```python
from build123d import *

# Parameters (mm, degrees)
SKETCH1_R           = 68.2625
SKETCH1_R_2         = 26.9875
BOSS_EXTRUDE1_DEPTH = 3.175


with BuildPart() as part:
    # Sketch1 → Boss-Extrude1 (new body)
    with BuildSketch(Plane.XY):
        Circle(SKETCH1_R)
        Circle(SKETCH1_R_2, mode=Mode.SUBTRACT)
        with BuildLine():
            ThreePointArc((-13.407442068, 58.659886532), (-30.0863, 52.111000212), (-44.097230886, 40.941128696))
            ThreePointArc((-44.097230886, 40.941128696), (-43.930699534, 36.454089884), (-39.443660721, 36.620621236))
            ThreePointArc((-39.443660721, 36.620621236), (-26.9113, 46.611738898), (-11.992557932, 52.46952282))
            ThreePointArc((-11.992557932, 52.46952282), (-9.604818144, 56.272146744), (-13.407442068, 58.659886532))
        make_face(mode=Mode.SUBTRACT)
        with BuildLine():
            ThreePointArc((39.443660721, 36.620621236), (26.9113, 46.611738898), (11.992557932, 52.46952282))
            ThreePointArc((11.992557932, 52.46952282), (9.604818144, 56.272146744), (13.407442068, 58.659886532))
            ThreePointArc((13.407442068, 58.659886532), (30.0863, 52.111000212), (44.097230886, 40.941128696))
            ThreePointArc((44.097230886, 40.941128696), (43.930699534, 36.454089884), (39.443660721, 36.620621236))
        make_face(mode=Mode.SUBTRACT)
        with BuildLine():
            ThreePointArc((51.436218653, -15.848901585), (53.8226, 0), (51.436218653, 15.848901585))
            ThreePointArc((51.436218653, 15.848901585), (53.535517678, 19.81805686), (57.504672954, 17.718757836))
            ThreePointArc((57.504672954, 17.718757836), (60.1726, 0), (57.504672954, -17.718757836))
            ThreePointArc((57.504672954, -17.718757836), (53.535517678, -19.81805686), (51.436218653, -15.848901585))
        make_face(mode=Mode.SUBTRACT)
        with BuildLine():
            ThreePointArc((11.992557932, -52.46952282), (26.9113, -46.611738898), (39.443660721, -36.620621236))
            ThreePointArc((39.443660721, -36.620621236), (43.930699534, -36.454089884), (44.097230886, -40.941128696))
            ThreePointArc((44.097230886, -40.941128696), (30.0863, -52.111000212), (13.407442068, -58.659886532))
            ThreePointArc((13.407442068, -58.659886532), (9.604818144, -56.272146744), (11.992557932, -52.46952282))
        make_face(mode=Mode.SUBTRACT)
        with BuildLine():
            ThreePointArc((-39.443660721, -36.620621236), (-26.9113, -46.611738898), (-11.992557932, -52.46952282))
            ThreePointArc((-11.992557932, -52.46952282), (-9.604818144, -56.272146744), (-13.407442068, -58.659886532))
            ThreePointArc((-13.407442068, -58.659886532), (-30.0863, -52.111000212), (-44.097230886, -40.941128696))
            ThreePointArc((-44.097230886, -40.941128696), (-43.930699534, -36.454089884), (-39.443660721, -36.620621236))
        make_face(mode=Mode.SUBTRACT)
        with BuildLine():
            ThreePointArc((-51.436218653, 15.848901585), (-53.8226, 0), (-51.436218653, -15.848901585))
            ThreePointArc((-51.436218653, -15.848901585), (-53.535517678, -19.81805686), (-57.504672954, -17.718757836))
            ThreePointArc((-57.504672954, -17.718757836), (-60.1726, 0), (-57.504672954, 17.718757836))
            ThreePointArc((-57.504672954, 17.718757836), (-53.535517678, 19.81805686), (-51.436218653, 15.848901585))
        make_face(mode=Mode.SUBTRACT)
    extrude(amount=BOSS_EXTRUDE1_DEPTH)


solid = part.part
```
For this review, take the finished solid that the model builds, in its own axes (mm). Round coordinates to 2 decimals unless told otherwise and drop trailing zeros. Write each loop counter-clockwise with the first axis right and the second up, starting at its lowest first coordinate (ties: lowest second). Pieces come first, ordered by that corner, then holes. Notation, with made-up numbers: (63, -17) - (68, -17) arc R11 cw to (68, 1) - close; hole circle Ø6 at (-7, -36). An arc over 180 degrees is marked (long way). Use CSV: the item, a comma, the result in double quotes.
1) Add section C-C on z = 0.6. Count the separate pieces of the cut face and the enclosed holes in it, and give its area (3 significant figures).
Conclusion:
separate pieces,"1"
enclosed holes,"7"
area,"10,900 mm^2"
2) Wall thickness on line 1 along Y through (x, z) = (0, 1.8); line 2 along X through (y, z) = (6, 2.7); line 3 along X through (y, z) = (-47.5, 0.75): over which ranges is each line inside the solid? List them lowest first. Write a range as from..to.
Conclusion:
line 1,"y = -68.26..-26.99, 26.99..68.26"
line 2,"x = -68..-59.87, -53.49..-26.31, 26.31..53.49, 59.87..68"
line 3,"x = -49.03..-36.94, -25.31..25.31, 36.94..49.03"
3) The part is to be moulded in two halves that separate along X. For faces 1 (the cylindrical face through (26.72, -46.72, 1.57)), 2 (the cylindrical face through (-68.196, 3.001, 1.565)), 3 (the flat face through (-1, -29, 3.175)), say which applies: pulls with the +X half, pulls with the -X half, needs draft (parallel to the pull), parting line crosses it, or undercut.
Conclusion:
face 1,"undercut"
face 2,"parting line crosses it"
face 3,"needs draft"
4) Add section A-A on x = 0. Write out the cut boundary in (y, z) (1 decimal), and give its area (3 significant figures).
Conclusion:
outline,"(-68.3, 0) - (-27, 0) - (-27, 3.2) - (-68.3, 3.2) - close; (27, 0) - (68.3, 0) - (68.3, 3.2) - (27, 3.2) - close"
area,"262 mm^2"
5) Add section D-D on y = 34. Write out the cut boundary in (x, z) (3 decimals).
Conclusion:
outline,"(-59.193, 0) - (59.193, 0) - (59.193, 3.175) - (-59.193, 3.175) - close"
6) Add section B-B on y = 0. Write out the cut boundary in (x, z) (1 decimal), and give its area (3 significant figures).
Conclusion:
outline,"(-68.3, 0) - (-60.2, 0) - (-60.2, 3.2) - (-68.3, 3.2) - close; (-53.8, 0) - (-27, 0) - (-27, 3.2) - (-53.8, 3.2) - close; (27, 0) - (53.8, 0) - (53.8, 3.2) - (27, 3.2) - close; (60.2, 0) - (68.3, 0) - (68.3, 3.2) - (60.2, 3.2) - close"
area,"222 mm^2"
7) Clearance check with flat-ended pins moving along their axes: pin 1 Ø1.5 at (y, z) = (-21, 2) entering from +X; pin 2 Ø1.5 at (x, z) = (24, 1) entering from +Y; pin 3 Ø1.5 at (x, z) = (36.5, 2) entering from +Y. State where each tip first meets the part, or that it passes through.
Conclusion:
pin 1,"stops at x = 65.19"
pin 2,"stops at y = 64.18"
pin 3,"stops at y = 58.15"
